For this review, take the finished solid that the model builds, in its own axes (mm). A direction names the side the tool comes from. Coordinates: 2 decimals unless noted, no trailing zeros. Loops run counter-clockwise (first coordinate to the right, second up) from the corner with the lowest first, then second, coordinate; pieces in that order, holes last. Notation, with made-up numbers: (81, 36) -> (107, 36) arc R22 cw to (107, 68) -> close; hole circle Ø11 at (18, -13.5). An arc over 180 degrees is marked (long way). Use a Markdown table: item, result.
from build123d import *

# Parameters (mm, degrees)
BOSS_EXTRUDE1_DEPTH = 8
SKETCH2_W           = 8
SKETCH2_H           = 70
BOSS_EXTRUDE2_DEPTH = 3
BOSS_EXTRUDE3_DEPTH = 8
SKETCH3_R           = 1.95
CUT_EXTRUDE1_DEPTH  = 5
BOSS_EXTRUDE4_DEPTH = 8


with BuildPart() as part:
    # Model → Boss-Extrude1 (new body)
    with BuildSketch(Plane.XY):
        Polygon((17.413449519, 34.221897901), (17.762016684, 34.366278619), (17.906397402, 34.714845785), (17.906397402, 47.038542874), (17.756302008, 47.793113579), (17.328872656, 48.432811545), (16.689176573, 48.860240897), (15.934604921, 49.010334408), (0, 49.010334408), (0, 0), (18.712346706, 0), (18.997450676, 0.090807901), (19.177512865, 0.329780152), (19.186191134, 0.62886938), (19.020288696, 0.877880987), (15.349128974, 4.028884693), (15.088389968, 4.05856896), (14.948683096, 3.83642518), (14.948683096, 1.933808007), (4.297410215, 1.933808007), (3.945501494, 2.087854221), (3.823764179, 2.426754717), (3.938850818, 2.765655441), (4.297410215, 2.919701654), (12.46281762, 2.919701654), (12.846572657, 2.997178421), (13.159951014, 3.208463791), (13.371237094, 3.521841448), (13.448713387, 3.905595539), (13.448713387, 38.433111261), (14.948709154, 38.433111261), (15.975012914, 34.783087212), (16.33877785, 34.373913238), (16.864740741, 34.221897901), align=None)
    extrude(amount=BOSS_EXTRUDE1_DEPTH)

    # Sketch2 → Boss-Extrude2 (add)
    with BuildSketch(Plane.ZY):
        with Locations((4, 24.505167204)):
            Rectangle(SKETCH2_W, SKETCH2_H)
    extrude(amount=BOSS_EXTRUDE2_DEPTH)

    # Sketch4 → Boss-Extrude3 (add)
    with BuildSketch(Plane.XY.offset(8)):
        Polygon((0, 59.505167204), (3.967302461, 49.010334408), (0, 49.010334408), align=None)
        Polygon((0, 0), (0, -10.494832796), (3.967302461, 0), align=None)
    extrude(amount=-BOSS_EXTRUDE3_DEPTH)

    # Sketch3 → Cut-Extrude1 (cut)
    with BuildSketch(Plane.ZY.offset(3)):
        with Locations((4, 49.555167204)):
            Circle(SKETCH3_R)
        with Locations((4, -0.544832796)):
            Circle(SKETCH3_R)
    extrude(amount=-CUT_EXTRUDE1_DEPTH, mode=Mode.SUBTRACT)

    # Sketch5 → Boss-Extrude4 (add)
    with BuildSketch(Plane.XY.offset(8)):
        Polygon((14.948709154, 38.433111261), (15.314043683, 37.133808007), (13.448713387, 37.133808007), (13.448713387, 38.433111261), align=None)
    extrude(amount=-BOSS_EXTRUDE4_DEPTH)


solid = part.part
(1) For pin 1 Ø4.5 at (y, z) = (-0.5, 4) entering from -X; pin 2 Ø2 at (y, z) = (14.5, 1.5) entering from +X; pin 3 Ø2.5 at (y, z) = (-0.54, 4) entering from -X; pin 4 Ø0.6 at (x, z) = (15, 5) entering from -Y, all flat-tipped, find the tip position at first contact; note any pin that passes through.
Found:
| item | result |
|---|---|
| pin 1 | stops at x = -3 |
| pin 2 | stops at x = 13.45 |
| pin 3 | stops at x = 2 |
| pin 4 | stops at y = 0 |
(2) Take a section at B-B on y = 16. Write out the cut boundary in (x, z), plus the area to 3 significant figures.
Found:
| item | result |
|---|---|
| outline | (-3, 0) -> (13.45, 0) -> (13.45, 8) -> (-3, 8) -> close |
| area | 132 mm^2 |
(3) For line 1 along Y through (x, z) = (-1.6, 4); line 2 along Y through (x, z) = (7.75, 7.5); line 3 along X through (y, z) = (13.5, 2), list the stretches that pass through material, from the lowest coordinate up.
Found:
| item | result |
|---|---|
| line 1 | y = -10.49 to -2.49, 1.41 to 47.61, 51.51 to 59.51 |
| line 2 | y = 0 to 1.93, 2.92 to 49.01 |
| line 3 | x = -3 to 13.45 |
(4) For faces 5 (the face through (2, 50, 4)), 6 (the face through (10, 49.01, 4)), 7 (the face through (11, 0, 4)), list the 3-axis set-ups (+Z, -Z, +X, -X, +Y, -Y) from which the entire face can be reached by the end or side of a thin tool; tool diameter is ignored.
Found:
| item | result |
|---|---|
| face 5 | -X |
| face 6 | +Z, -Z, +X, +Y |
| face 7 | +Z, -Z, +X, -Y |
(5) Mouldability with a two-part tool opening along Z and no side actions: class faces 1 (the face through (-0.54, 51.49, 3.75)), 2 (the face through (2, -1, 4)), 3 (the face through (14.949, 3, 4)), 4 (the face through (6, 25, 0)) as pulls with the +Z half, pulls with the -Z half, needs draft (parallel to the pull), parting line crosses it, or undercut.
Found:
| item | result |
|---|---|
| face 1 | undercut |
| face 2 | undercut |
| face 3 | needs draft |
| face 4 | pulls with the -Z half |
(6) Take a section at A-A on y = 46. Write out the cut boundary in (x, z), plus the area to 3 significant figures.
Found:
| item | result |
|---|---|
| outline | (-3, 0) -> (17.91, 0) -> (17.91, 8) -> (-3, 8) -> close |
| area | 167 mm^2 |
